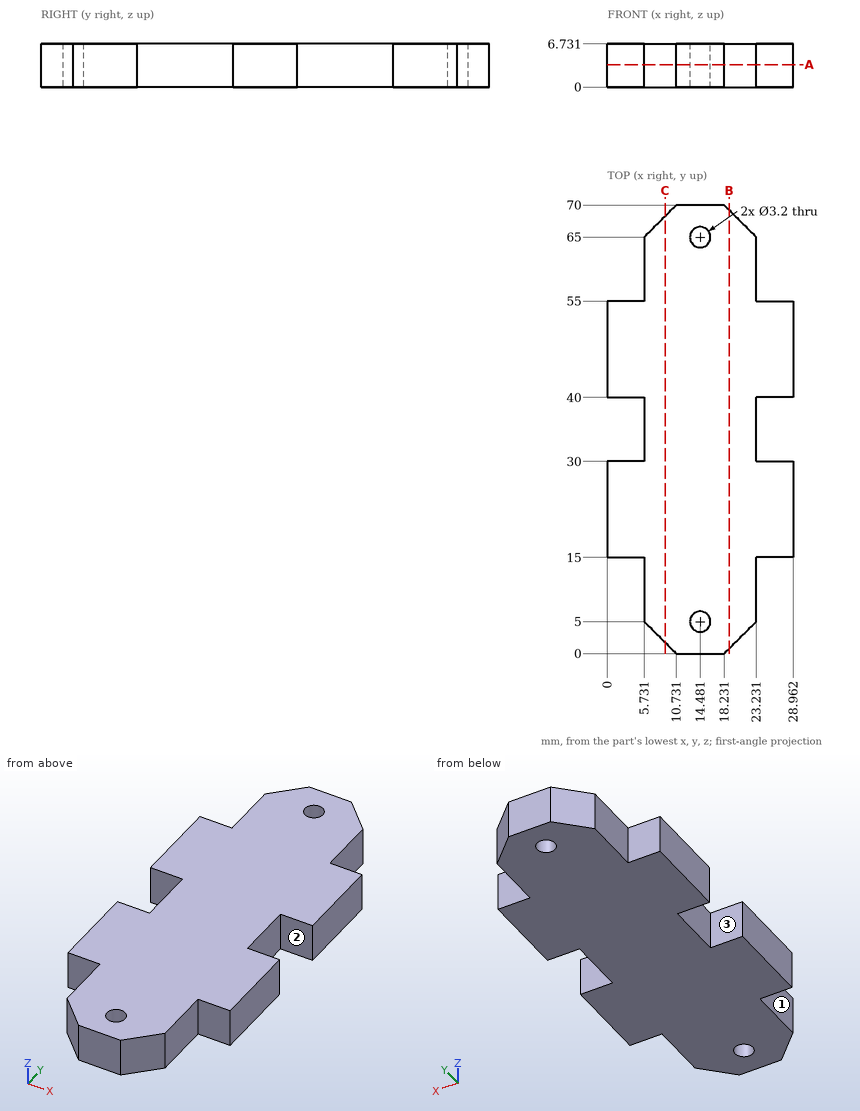
Study the drawing (mm; zero at the part's minimum x, y, z) and answer. A direction names the side the tool comes from. Round coordinates to 2 decimals unless told otherwise and drop trailing zeros. Write each loop counter-clockwise with the first axis right and the second up, starting at its lowest first coordinate (ties: lowest second). Pieces come first, ordered by that corner, then holes.
Q1. Find section B-B on x = 19. Determine the outline of the cut face in (y, z).
Values:
outline: (0.77, 0) - (69.23, 0) - (69.23, 6.73) - (0.77, 6.73) - close
Q2. Flat-ended cylindrical pins translate along their axes: P1, Ø3, axis at x = 26.5, z = 3.5, coming from the -Y side; P2, Ø2, axis at y = 8.5, z = 4.5, coming from the -X side; P3, Ø1, axis at y = 33.5, z = 6, coming from the +X side. Find the tip coordinate at first contact, or state that the pin passes through.
Values:
P1: stops at y = 15
P2: stops at x = 5.73
P3: stops at x = 23.23
Q3. Straight lines are drawn through the part: line 1 (Y direction, x = 25, z = 0.5); line 2 (X direction, y = 65, z = 3.25); line 3 (Y direction, x = 15.25, z = 3.25). For each, find the intervals that lie inside material, in ascending order.
Values:
line 1: y = 15 to 30, 40 to 55
line 2: x = 5.73 to 12.88, 16.08 to 23.23
line 3: y = 0 to 3.6, 6.4 to 63.6, 66.4 to 70
Q4. Find section A-A on z = 3.5. Determine the outline of the cut face in (x, y).
Values:
outline: (0, 15) - (5.73, 15) - (5.73, 5) - (10.73, 0) - (18.23, 0) - (23.23, 5) - (23.23, 15) - (28.96, 15) - (28.96, 30) - (23.23, 30) - (23.23, 40) - (28.96, 40) - (28.96, 55) - (23.23, 55) - (23.23, 65) - (18.23, 70) - (10.73, 70) - (5.73, 65) - (5.73, 55) - (0, 55) - (0, 40) - (5.73, 40) - (5.73, 30) - (0, 30) - close; hole circle Ø3.2 at (14.48, 5); hole circle Ø3.2 at (14.48, 65)
Q5. A tool of negligible diameter and unlimited length cuts with its end or side. For the marked faces 1, 2 and 3, from which of +Z, -Z, +X, -X, +Y, -Y can it reach the whole face along a straight path? Write none if from no direction.
Values:
face 1: +Z, -Z, -X, -Y
face 2: +Z, -Z, +X
face 3: +Z, -Z, -X
Q6. Find section C-C on x = 9. Determine the outline of the cut face in (y, z).
Values:
outline: (1.73, 0) - (68.27, 0) - (68.27, 6.73) - (1.73, 6.73) - close
